CAD build for the part. Positions are in the model's coordinates, mm. A direction names the side the tool comes from. Give positions to 0.01 mm unless a question says otherwise; leave off trailing zeros. Write each loop counter-clockwise with the first axis right and the second up, starting at its lowest first coordinate (ties: lowest second). Pieces come first, ordered by that corner, then holes. Notation, with made-up numbers: (46, 73.5) -> (64, 73.5) arc R22 cw to (64, 80.5) -> close; hole circle Ø8 at (72, -17). An arc over 180 degrees is marked (long way). Answer as a JSON object with one key per item and string values.
Autodesk Inventor part; units mm, degrees
ref_plane "YZ Plane" through (0, 0, 0) normal (1, 0, 0) x (0, 1, 0)
ref_plane "XZ Plane" through (0, 0, 0) normal (0, 1, 0) x (-1, 0, 0)
ref_plane "XY Plane" through (0, 0, 0) normal (0, 0, 1) x (1, 0, 0)
sketch "Sketch1" plane through (0, 0, 0) normal (0, 1, 0) x (-1, 0, 0)
  circle A0 centre (0, 0) radius 4
  circle A1 centre (0, 0) radius 5
  circle A2 centre (0, 0) radius 1
  circle A3 centre (0, 0) radius 1.5
  dimension "d0" = 8
  dimension "d1" = 10
  dimension "d2" = 2
  dimension "d3" = 3
extrude "Extrusion1" add sketch "Sketch1" along normal blind 10 contours A1
extrude "Extrusion2" add sketch "Sketch1" along normal blind 4 contours A0 | A3
extrude "Extrusion3" add sketch "Sketch1" against normal blind 8 contours A3
thread "Thread1"
1) Mould opens along Z. For faces 3 (the cylindrical face through (0, -2, -1)), 4 (the flat face through (1.2, 0, 1.2)), 5 (the cylindrical face through (1.5, -3.94, 0.07)) say: released by +Z, released by -Z, zero draft, split by the parting line, or undercut.
Model answer:
{"face 3": "undercut", "face 4": "zero draft", "face 5": "split by the parting line"}
2) Slice it at C-C (y = 9). List the corners of the cut face in (x, z), then the cut area to 3 significant figures.
Model answer:
{"outline": "circle Ø10 at (0, 0); hole circle Ø8 at (0, 0)", "area": "28.3 mm2"}
3) Pin check, flat tips, straight feed: pin 1 (3 mm diameter, centred on x = -2.5, y = -4.5, fed in from -Z); pin 2 (3 mm diameter, centred on x = -1, z = -1, fed in from +Y); pin 3 (4 mm diameter, centred on x = 1.5, y = -3.5, fed in from +Z). Stop position of each tip, or through.
Model answer:
{"pin 1": "stops at z = -1.12", "pin 2": "stops at y = 4", "pin 3": "stops at z = 1.5"}
4) 3-axis set-ups, long thin cutter, end or side, ignore diameter. For faces 1 (the cylindrical face through (1.08, 4.93, 4.88)), 2 (the cylindrical face through (0.867, 6.958, 3.905)): which of +Z, -Z, +X, -X, +Y, -Y reach the whole face in a straight line?
Model answer:
{"face 1": "+Y, -Y", "face 2": "+Y"}
5) Slice it at B-B (x = 0). List the corners of the cut face in (y, z).
Model answer:
{"outline": "(-8, -1.5) -> (0, -1.5) -> (0, -5) -> (10, -5) -> (10, -4) -> (4, -4) -> (4, -1) -> (-8, -1) -> close; (-8, 1) -> (4, 1) -> (4, 4) -> (10, 4) -> (10, 5) -> (0, 5) -> (0, 1.5) -> (-8, 1.5) -> close"}
6) Slice it at D-D (x = 2.75). List the corners of the cut face in (y, z).
Model answer:
{"outline": "(0, -4.18) -> (10, -4.18) -> (10, -2.9) -> (4, -2.9) -> (4, 2.9) -> (10, 2.9) -> (10, 4.18) -> (0, 4.18) -> close"}
7) Slice it at A-A (z = 0). List the corners of the cut face in (x, y), then the cut area to 3 significant figures.
Model answer:
{"outline": "(-5, 0) -> (-1.5, 0) -> (-1.5, -8) -> (-1, -8) -> (-1, 4) -> (-4, 4) -> (-4, 10) -> (-5, 10) -> close; (1, -8) -> (1.5, -8) -> (1.5, 0) -> (5, 0) -> (5, 10) -> (4, 10) -> (4, 4) -> (1, 4) -> close", "area": "52.0 mm2"}
8) Wall check: probe 1 along Z at (x, y) = (0, 7.35); probe 2 along Z at (x, y) = (0, -3.25); probe 3 along Y at (x, z) = (2.75, 1.5). Give the ranges that are in metal, low to high.
Model answer:
{"probe 1": "z = -5 to -4, 4 to 5", "probe 2": "z = -1.5 to -1, 1 to 1.5", "probe 3": "y = 0 to 4"}
